The figure shows three views and two pictorial views of one solid part (mm, origin at its lowest corner). Answer the questions. Coordinates: 2 decimals unless noted, no trailing zeros. Loops run counter-clockwise (first coordinate to the right, second up) from the corner with the lowest first, then second, coordinate; pieces in that order, holes last. Notation, with made-up numbers: (-32.75, 88.25) -> (-18.75, 88.25) arc R13 cw to (-18.75, 104.25) -> close; hole circle Ø8 at (0.25, -4). An arc over 180 degrees is marked (long way). Use a Markdown table: item, result. Add a question column.
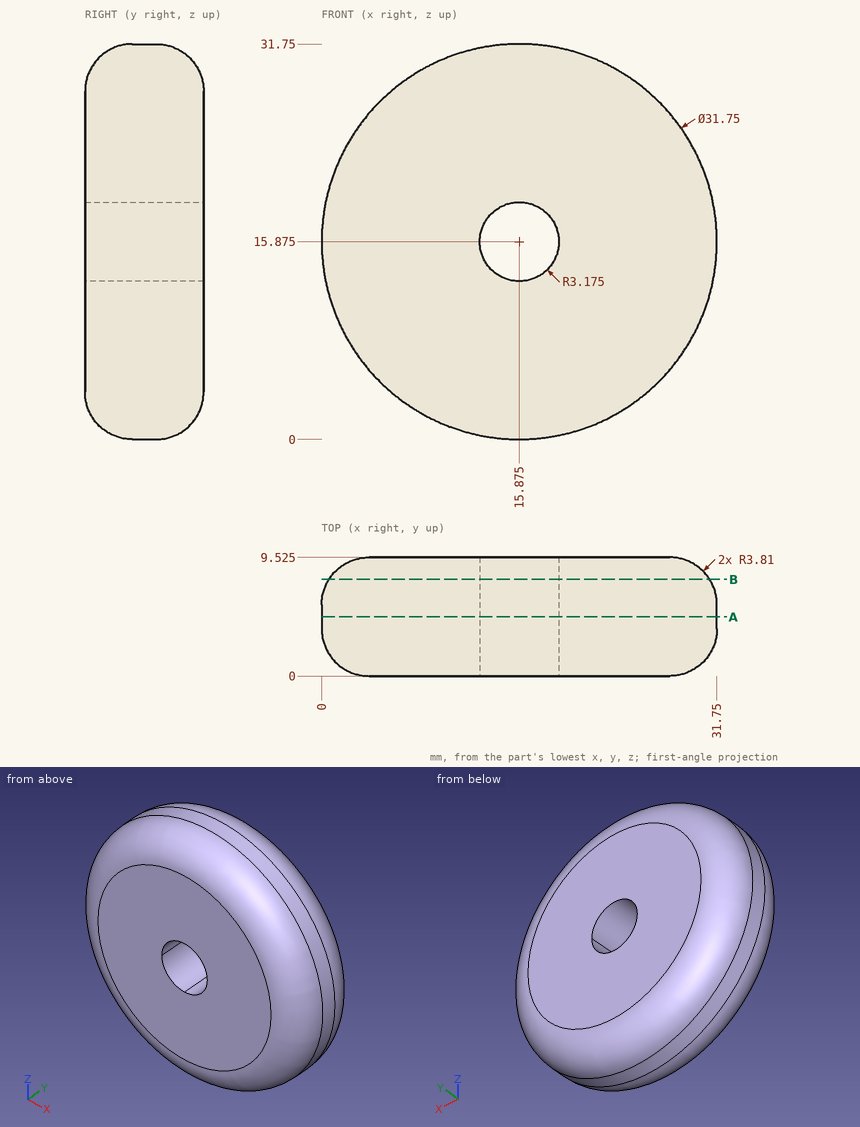
Item 1: Find the intervals of material crossed by probe 1 along Z at (x, y) = (13.5, 7); probe 2 along X at (y, z) = (5.75, 18.5); probe 3 along X at (y, z) = (4, 14.5), in increasing order.
Item 2: Given pin 1 (1 mm diameter, centred on x = 8.5, y = 6.5, fed in from +Z); pin 2 (1 mm diameter, centred on y = 3.5, z = 21, fed in from +X); pin 3 (3 mm diameter, centred on y = 5, z = 23, fed in from +X), each flat-ended and moving along its own axis, determine where each tip first touches the part or whether it passes through.
Item 3: Section A-A (y = 4.75) is taken. Determine the outline of the cut face in (x, z) (3 decimals), then the cut area to 3 significant figures.
Item 4: Section B-B (y = 7.75) is taken. Determine the outline of the cut face in (x, z) (3 decimals), then the cut area to 3 significant figures.
Output:
| question | item | result |
|---|---|---|
| 1 | probe 1 | z = 0.4 to 13.77, 17.98 to 31.35 |
| 1 | probe 2 | x = 0.22 to 14.09, 17.66 to 31.53 |
| 1 | probe 3 | x = 0.06 to 13.01, 18.74 to 31.69 |
| 2 | pin 1 | stops at z = 30.11 |
| 2 | pin 2 | stops at x = 31.05 |
| 2 | pin 3 | stops at x = 30.72 |
| 3 | outline | circle Ø31.75 at (15.875, 15.875); hole circle Ø6.35 at (15.875, 15.875) |
| 3 | area | 760 mm2 |
| 4 | outline | circle Ø30.572 at (15.875, 15.875); hole circle Ø6.35 at (15.875, 15.875) |
| 4 | area | 702 mm2 |
